Read the model definition and answer for the solid it produces. Units are mm, in the model's axes. A direction names the side the tool comes from. Round coordinates to 2 decimals unless told otherwise and drop trailing zeros. Order: outer loops, then holes, each group sorted by start corner. A loop starts at its lowest first (then second) coordinate and runs counter-clockwise, first axis right, second up. Notation, with made-up numbers: (22.25, 18) -> (36.25, 18) arc R15 cw to (36.25, 41) -> close; hole circle Ø6 at (-33.5, -24). An arc over 180 degrees is marked (long way). Use a Markdown table: item, result. Add a question column.
1. Section B-B, the plane x = -5.5 is taken. Give the vertices of the cut face in (y, z).
2. The mould has two halves that part along Z. Classify faces 1 (the face through (-76.307, -0.74, 34.883)), 2 (the face through (-26, -1.5, 20)), 3 (the face through (-24.717, -0.74, 13.418)), 4 (the face through (-90, -0.7, 37.4)): +Z half, -Z half, draft (parallel to the pull), parting line (faces both ways), or undercut.
3. Section A-A, the plane y = -0.4 is taken. Give the number of separate pieces and of enclosed holes in the cut face, then the cut area to 3 significant figures.
4. Given pin 1 (3 mm diameter, centred on x = -54.5, z = 28.5, fed in from +Y); pin 2 (0.8 mm diameter, centred on x = -16.5, y = -0.5, fed in from +Z), each flat-ended and moving along its own axis, determine where each tip first touches the part or whether it passes through.
5. Consider L1, parallel to X at y = -1.1, z = 27; L2, parallel to Z at x = -19.78, y = -0.7; L3, parallel to Z at x = -26.78, y = -0.55. Determine where each line is inside the solid, lowest interval first. Write a range as [from, to].
6. For faces 5 (the face through (22.71, -0.74, 34.85)), 6 (the face through (-26, 0, 20)), determine the directions among +Z, -Z, +X, -X, +Y, -Y from which every point of the face is accessible in a straight line to the end or side of a thin tool.
Autodesk Inventor part; units mm, degrees
ref_plane "YZ Plane" through (0, 0, 0) normal (1, 0, 0) x (0, 1, 0)
ref_plane "XZ Plane" through (0, 0, 0) normal (0, 1, 0) x (-1, 0, 0)
ref_plane "XY Plane" through (0, 0, 0) normal (0, 0, 1) x (1, 0, 0)
sketch "Sketch1" plane through (0, 0, 0) normal (0, 1, 0) x (-1, 0, 0)
  line L0 (-0.4496, 29.8144) -> (-0.4496, -0.0878)
  line L1 (54.0096, -0.0338) -> (54.0096, 29.8144)
  line L2 (53.5706, 0) -> (53.6221, -0.0838)
  line L3 (53.56, 0) -> (53.5706, 0)
  line L4 (53.56, -0.0837) -> (53.56, 0)
  line L5 (-0.0106, 0) -> (-0.0621, -0.0838)
  line L6 (-0.8993, -0.0972) -> (-0.0106, 0)
  line L7 (53.5706, 0) -> (54.4593, -0.0972)
  line L8 (0, 0) -> (0, -0.0837)
  line L9 (-0.0106, 0) -> (0, 0)
  line L10 (0, 0) -> (53.56, 0)
  line L11 (53.7094, 29.5089) -> (53.5853, 29.9994)
  line L12 (53.56, 29.512) -> (53.7094, 29.5089)
  line L13 (53.56, 30) -> (53.56, 29.512)
  line L14 (-0.1494, 29.5089) -> (-0.0253, 29.9994)
  line L15 (-0.8993, 29.4222) -> (-0.1494, 29.5089)
  line L16 (0, 29.512) -> (0, 30)
  line L17 (-0.1494, 29.5089) -> (0, 29.512)
  line L18 (53.7094, 29.5089) -> (54.4593, 29.4222)
  line L19 (0, 29.512) -> (53.56, 29.512)
  circle A0 centre (26.78, 15) radius 2.6
  circle A1 centre (84.5793, 29) radius 2.6
  circle A2 centre (-31.0193, 29) radius 3.6
  circle A3 centre (91.5793, 29) radius 1.05
  circle A4 centre (84.5793, 36) radius 1.05
  circle A5 centre (84.5793, 22) radius 1.05
  circle A6 centre (77.5793, 29) radius 1.05
  circle A7 centre (-38.0193, 29) radius 1.05
  circle A8 centre (-31.0193, 36) radius 1.05
  circle A9 centre (-31.0193, 22) radius 1.05
  circle A10 centre (-24.0193, 29) radius 1.05
  circle A11 centre (19.78, 15) radius 1.05
  circle A12 centre (26.78, 22) radius 1.05
  circle A13 centre (33.78, 15) radius 1.05
  circle A14 centre (26.78, 8) radius 1.05
  line L20 (53.5853, 29.9994) -> (53.56, 30)
  line L21 (53.6221, -0.0838) -> (53.56, -0.0837)
  line L22 (-0.0621, -0.0838) -> (-0.8993, -0.0972)
  line L23 (-0.0253, 29.9994) -> (-0.8993, 29.4222)
  line L24 (77.602, 36.0383) -> (74.975, 33.6954)
  line L25 (74.975, 33.6954) -> (72.272, 31.7856)
  line L26 (72.272, 31.7856) -> (69.4931, 30.3089)
  line L27 (69.4931, 30.3089) -> (66.6383, 29.2653)
  line L28 (66.6383, 29.2653) -> (63.7075, 28.6549)
  line L29 (63.7075, 28.6549) -> (60.7007, 28.4776)
  line L30 (60.7007, 28.4776) -> (57.618, 28.7333)
  line L31 (57.618, 28.7333) -> (54.4593, 29.4222)
  line L32 (54.4593, -0.0972) -> (53.6221, -0.0838)
  line L33 (-40.5487, 25.8824) -> (-39.4527, 22.5565)
  line L34 (-39.4527, 22.5565) -> (-38.1807, 19.4832)
  line L35 (-38.1807, 19.4832) -> (-36.7234, 16.6331)
  line L36 (-36.7234, 16.6331) -> (-35.0805, 14.0064)
  line L37 (-35.0805, 14.0064) -> (-33.2522, 11.6029)
  line L38 (-33.2522, 11.6029) -> (-31.2384, 9.4228)
  line L39 (-31.2384, 9.4228) -> (-29.0391, 7.4659)
  line L40 (-29.0391, 7.4659) -> (-26.6543, 5.7324)
  line L41 (-26.6543, 5.7324) -> (-24.0841, 4.2221)
  line L42 (-24.0841, 4.2221) -> (-21.3284, 2.9352)
  line L43 (-21.3284, 2.9352) -> (-18.3872, 1.8715)
  line L44 (-18.3872, 1.8715) -> (-15.2606, 1.0312)
  line L45 (-15.2606, 1.0312) -> (-11.9485, 0.4141)
  line L46 (-11.9485, 0.4141) -> (-8.4509, 0.0204)
  line L47 (-8.4509, 0.0204) -> (-4.7678, -0.1501)
  line L48 (-4.7678, -0.1501) -> (-0.8993, -0.0972)
  line L49 (0, 30) -> (-0.0253, 29.9994)
  line L50 (54.4593, -0.0972) -> (58.3278, -0.1501)
  line L51 (58.3278, -0.1501) -> (62.0109, 0.0204)
  line L52 (62.0109, 0.0204) -> (65.5085, 0.4141)
  line L53 (65.5085, 0.4141) -> (68.8206, 1.0312)
  line L54 (68.8206, 1.0312) -> (71.9472, 1.8715)
  line L55 (71.9472, 1.8715) -> (74.8884, 2.9352)
  line L56 (74.8884, 2.9352) -> (77.6441, 4.2221)
  line L57 (77.6441, 4.2221) -> (80.2143, 5.7324)
  line L58 (80.2143, 5.7324) -> (82.5991, 7.4659)
  line L59 (82.5991, 7.4659) -> (84.7984, 9.4228)
  line L60 (84.7984, 9.4228) -> (86.8122, 11.6029)
  line L61 (86.8122, 11.6029) -> (88.6405, 14.0064)
  line L62 (88.6405, 14.0064) -> (90.2834, 16.6331)
  line L63 (90.2834, 16.6331) -> (91.7407, 19.4832)
  line L64 (91.7407, 19.4832) -> (93.0127, 22.5565)
  line L65 (93.0127, 22.5565) -> (94.1087, 25.8824)
  line L66 (54.4593, 29.4222) -> (53.5853, 29.9994)
  line L67 (-0.8993, 29.4222) -> (-4.058, 28.7333)
  line L68 (-4.058, 28.7333) -> (-7.1407, 28.4776)
  line L69 (-7.1407, 28.4776) -> (-10.1475, 28.6549)
  line L70 (-10.1475, 28.6549) -> (-13.0783, 29.2653)
  line L71 (-13.0783, 29.2653) -> (-15.9331, 30.3089)
  line L72 (-15.9331, 30.3089) -> (-18.712, 31.7856)
  line L73 (-18.712, 31.7856) -> (-21.415, 33.6954)
  line L74 (-21.415, 33.6954) -> (-24.042, 36.0383)
  line L75 (0, -0.0837) -> (-0.0621, -0.0838)
  line L76 (53.56, 30) -> (0, 30)
  arc A15 (-24.042, 36.0383) -> (-40.5487, 25.8824) centre (-31.0892, 28.9999) ccw
  arc A16 (94.1087, 25.8824) -> (77.602, 36.0383) centre (84.6492, 28.9999) ccw
  line L77 (53.56, -0.0837) -> (0, -0.0837)
  line L78 (54.4593, 29.4222) -> (54.4593, -0.0972)
  line L79 (-0.8993, -0.0972) -> (-0.8993, 29.4222)
  line L80 (53.56, 0) -> (53.56, 30)
  line L81 (0, 30) -> (0, 0)
  point P0 (0, 0)
extrude "Extrusion1" add sketch "Sketch1" against normal blind 1.5 contours L15 L17 L81 L9 L6 L0 | L0 L6 L79 L15 | L79 L48 L47 L46 L45 L44 L43 L42 L41 L40 L39 L38 L37 L36 L35 L34 L33 A15 L74 L73 L72 L71 L70 L69 L68 L67 | L19 L80 L10 L81 | L12 L18 L78 L7 L3 L80 | L31 L30 L29 L28 L27 L26 L25 L24 A16 L65 L64 L63 L62 L61 L60 L59 L58 L57 L56 L55 L54 L53 L52 L51 L50 L78
extrude "Extrusion2" add sketch "Sketch1" against normal blind 1.5 contours L6 L5 L22 | L9 L8 L75 L5 | L10 L4 L77 L8 | L3 L2 L21 L4 | L7 L32 L2
sketch "Sketch2" plane through (0, 0, 0) normal (0, 1, 0) x (1, 0, 0)
  line L0 (-54.4593, -29.4222) -> (-54.4593, 0.0972)
  line L1 (0.8993, 0.0972) -> (0.8993, -29.4222)
  point P0 (0, 0)
properties part number "axis_21_bottom_frame"
Verdict:
| question | item | result |
|---|---|---|
| 1 | outline | (-1.5, -0.08) -> (0, -0.08) -> (0, 29.51) -> (-1.5, 29.51) -> close |
| 2 | face 1 | +Z half |
| 2 | face 2 | draft |
| 2 | face 3 | undercut |
| 2 | face 4 | parting line |
| 3 | separate pieces | 1 |
| 3 | enclosed holes | 15 |
| 3 | area | 3,720 mm2 |
| 4 | pin 1 | stops at y = 0 |
| 4 | pin 2 | stops at z = 29.51 |
| 5 | L1 | x = [-94.41, -86.24], [-82.92, 28.03], [34.01, 40.85] |
| 5 | L2 | z = [-0.08, 13.95], [16.05, 29.51] |
| 5 | L3 | z = [-0.08, 6.95], [9.05, 12.4], [17.6, 20.95], [23.05, 29.51] |
| 6 | face 5 | +Z, +Y, -Y |
| 6 | face 6 | +Z, -Z, +X, -X, +Y |
